```python
from build123d import *

# Parameters (mm, degrees)
F0_W     = 600
F0_H     = 900
F1_DEPTH = 25
F2_W     = 550
F2_H     = 450
F3_DEPTH = 50.001
F4_W     = 500
F4_H     = 400
F5_DEPTH = 50.001


with BuildPart() as f1:
    # F0 (on Right) → F1 (new body, symmetric)
    with BuildSketch(Plane.YZ):
        Rectangle(F0_W, F0_H)
    extrude(amount=F1_DEPTH, both=True)

    # F2 (on face) → F3 (cut, through all)
    with BuildSketch(Plane.YZ.offset(25)):
        with Locations((25, 225)):
            Rectangle(F2_W, F2_H)
    extrude(amount=-F3_DEPTH, mode=Mode.SUBTRACT)

    # F4 (on face) → F5 (cut, through all)
    with BuildSketch(Plane.YZ.offset(25)):
        with Locations((0, -250)):
            Rectangle(F4_W, F4_H)
    extrude(amount=-F5_DEPTH, mode=Mode.SUBTRACT)


solid = f1.part
```
Geometry: final body of the model. Coordinates: model frame, mm. A direction names the side the tool comes from. Coordinates: 2 decimals unless noted, no trailing zeros. Order: outer loops, then holes, each group sorted by start corner. A loop starts at its lowest first (then second) coordinate and runs counter-clockwise, first axis right, second up.
Item 1: Access query for faces 1 (the face through (0, -250, 222)), 2 (the face through (0, -275, 450)), 3 (the face through (0, -250, -253)). Directions: +Z, -Z, +X, -X, +Y, -Y. A direction counts if a zero-diameter tool reaches every point of the face in a straight line with its end or side. Return the directions, or none.
Answer:
face 1: +Z, +X, -X, +Y
face 2: +Z, +X, -X, +Y, -Y
face 3: -Z, +X, -X
Item 2: Material intervals for line 1 along Y through (x, z) = (4, -318.5); line 2 along Z through (x, y) = (-13, 234); line 3 along Z through (x, y) = (15, 274), sorted ascending.
Answer:
line 1: y = -300 to -250, 250 to 300
line 2: z = -50 to 0
line 3: z = -450 to 0
Item 3: Section query A-A (z = -65). Output: boundary loops of the cut face in (x, y), then the cut area to 3 significant figures.
Answer:
outline: (-25, -300) - (25, -300) - (25, -250) - (-25, -250) - close; (-25, 250) - (25, 250) - (25, 300) - (-25, 300) - close
area: 5,000 mm2
Item 4: Draft query along Y for faces 4 (the face through (25, -90, -31)), 5 (the face through (0, 250, -253)), 6 (the face through (0, -3, -50)), 7 (the face through (0, 300, -228)). Return one class per face: released by +Y, released by -Y, zero draft, split by the parting line, or undercut.
Answer:
face 4: zero draft
face 5: undercut
face 6: undercut
face 7: released by +Y
Item 5: Section query C-C (y = 132). Output: boundary loops of the cut face in (x, z).
Answer:
outline: (-25, -50) - (25, -50) - (25, 0) - (-25, 0) - close
Item 6: Contact query for flat-ended pins moving along their axis: P1, Ø12, axis at x = 11.5, y = -189.5, coming from the +Z side; P2, Ø15, axis at x = -3, y = 103, coming from the -Z side. Output: stop coordinate, or through.
Answer:
P1: stops at z = 0
P2: stops at z = -50
Item 7: Section query B-B (x = 10). Output: boundary loops of the cut face in (y, z), then the cut area to 3 significant figures.
Answer:
outline: (-300, -450) - (-250, -450) - (-250, -50) - (250, -50) - (250, -450) - (300, -450) - (300, 0) - (-250, 0) - (-250, 450) - (-300, 450) - close
area: 92,500 mm2
Item 8: Section query D-D (z = 271.5). Output: boundary loops of the cut face in (x, y).
Answer:
outline: (-25, -300) - (25, -300) - (25, -250) - (-25, -250) - close
